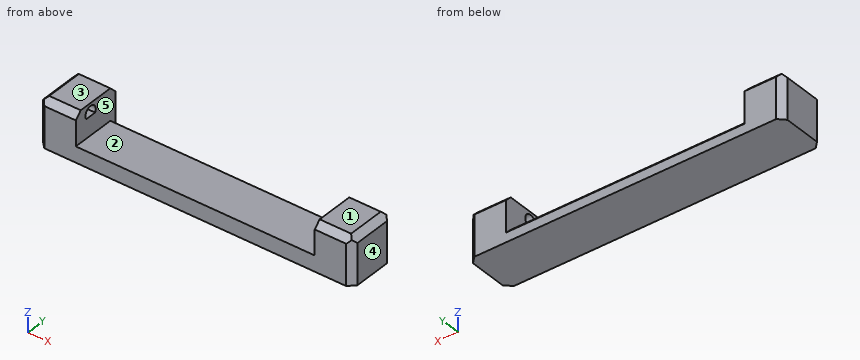
```python
from build123d import *

# Parameters (mm, degrees)
F0_W          = 100
F0_H          = 16
F1_DEPTH      = 3
F2_W          = 12
F2_H          = 16
F3_DEPTH      = 10
F4_SIZE       = 2
F5_SIZE       = 2
F6_SIZE       = 2
F8_DEPTH      = 84
F8_DEPTH_BACK = 8
F9_DEPTH      = 2


with BuildPart() as f1:
    # F0 (on Top) → F1 (new body)
    with BuildSketch(Plane.XY):
        Rectangle(F0_W, F0_H)
    extrude(amount=F1_DEPTH)

    # F2 (on face) → F3 (join)
    with BuildSketch(Plane.XY.offset(3)):
        with Locations((-44, 0)):
            Rectangle(F2_W, F2_H)
        with Locations((44, 0)):
            Rectangle(F2_W, F2_H)
    extrude(amount=F3_DEPTH)

    # F4
    f4_edges = [f1.edges().sort_by_distance(p)[0] for p in [
        (-50, 8, 6.5),
        (-50, 0, 13),
        (-50, -8, 6.5),
        (50, -8, 6.5),
        (50, 0, 13),
        (50, 8, 6.5),
    ]]
    chamfer(f4_edges, length=F4_SIZE)

    # F5
    f5_edges = [f1.edges().sort_by_distance(p)[0] for p in [
        (-43, -8, 13),
        (-43, 8, 13),
        (43, 8, 13),
        (43, -8, 13),
    ]]
    chamfer(f5_edges, length=F5_SIZE)

    # F6
    f6_edges = [f1.edges().sort_by_distance(p)[0] for p in [
        (0, 8, 3),
    ]]
    chamfer(f6_edges, length=F6_SIZE)

    # F9 (add): a face of the model
    f9_faces = [f1.faces().sort_by_distance(p)[0] for p in [
        (0, 0, 0),
    ]]
    extrude(f9_faces, amount=F9_DEPTH)


with BuildPart() as f8:
    # F7 (on face) → F8 (new body, two sides)
    with BuildSketch(Plane.YZ.offset(-38)) as f8_sk:
        with BuildLine():
            Line((-3.8466185313, 9), (-0.1533814687, 9))
            ThreePointArc((-0.1533814687, 9), (-2, 12.1), (-3.8466185313, 9))
        make_face()
    extrude(amount=F8_DEPTH)
    extrude(f8_sk.sketch, amount=-F8_DEPTH_BACK)


with BuildPart() as f1_1:
    add(f1.part)

    # F10: cut F8
    add(f8.part, mode=Mode.SUBTRACT)


solid = f1_1.part
```
For this review, take the finished solid that the model builds, in its own axes (mm). Face numbers are marked on the shaded views. A direction names the side the tool comes from. Give positions to 0.01 mm unless a question says otherwise; leave off trailing zeros. Write each loop counter-clockwise with the first axis right and the second up, starting at its lowest first coordinate (ties: lowest second). Pieces come first, ordered by that corner, then holes. Notation, with made-up numbers: M -1,78.5 L 3,78.5 A28 ccw 3,105.5 Z; hole C 61,41 d9. An arc over 180 degrees is marked long. Answer as CSV lines item,"result".
1. Consider section D-D, the plane y = 2.75. Write out the cut boundary in (x, z).
Findings:
outline,"M -50,-2 L 50,-2 L 50,11 L 48,13 L 38,13 L 38,3 L -38,3 L -38,13 L -48,13 L -50,11 Z"
2. Wall thickness on line 1 (X direction, y = -3, z = 6.25); line 2 (Y direction, x = 40.75, z = 10); line 3 (Z direction, x = -24, y = 2.25): over which ranges is each line inside the solid? List them lowest first.
Findings:
line 1,"x = -50 to -38, 38 to 50"
line 2,"y = -8 to -4.1, 0.1 to 8"
line 3,"z = -2 to 3"
3. For the marked faces 1 and 2, list the 3-axis set-ups (+Z, -Z, +X, -X, +Y, -Y) from which the entire face can be reached by the end or side of a thin tool; tool diameter is ignored.
Findings:
face 1,"+Z, +X, -X, +Y, -Y"
face 2,"+Z, +Y, -Y"
4. Consider section A-A, the plane z = 10. Write out the cut boundary in (x, y), then the cut area to 3 significant figures.
Findings:
outline,"M -50,-6 L -48,-8 L -38,-8 L -38,-4.1 L -46,-4.1 L -46,0.1 L -38,0.1 L -38,8 L -48,8 L -50,6 Z; M 38,-8 L 48,-8 L 50,-6 L 50,6 L 48,8 L 38,8 L 38,0.1 L 46,0.1 L 46,-4.1 L 38,-4.1 Z"
area,"309 mm2"
5. For pin 1 (4 mm diameter, centred on x = 18, y = 5.5, fed in from +Z), flat-tipped, find the tip position at first contact; note if it passes through.
Findings:
pin 1,"stops at z = 3"
6. Consider section C-C, the plane x = 29. Write out the cut boundary in (y, z).
Findings:
outline,"M -8,-2 L 8,-2 L 8,1 L 6,3 L -8,3 Z"
7. Consider section B-B, the plane y = -2. Write out the cut boundary in (x, z), then the cut area to 3 significant figures.
Findings:
outline,"M -50,-2 L 50,-2 L 50,11 L 48,13 L 38,13 L 38,12.1 L 46,12.1 L 46,9 L 38,9 L 38,3 L -38,3 L -38,9 L -46,9 L -46,12.1 L -38,12.1 L -38,13 L -48,13 L -50,11 Z"
area,"686 mm2"
8. Draft analysis for pull direction X (two halves, no side actions). For the marked faces 3, 4 and 5, state which applies: +X half, -X half, draft (parallel to the pull), parting line (faces both ways), or undercut.
Findings:
face 3,"draft"
face 4,"+X half"
face 5,"undercut"
